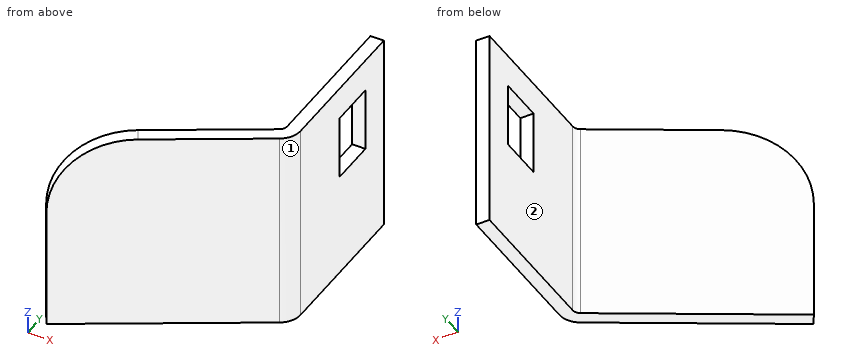
```python
from build123d import *

# Parameters (mm, degrees)
ODGI_CIE_BAZOWE1_DEPTH     = 76
ZAOKR_GLENIE1_R            = 30
WYTNIJ_WYCI_GNI_CIE1_REACH = 120.035
SZKIC2_W                   = 24.223008457
SZKIC2_H                   = 17.102544726


# Sheet-metal steps are written as plain solids
with BuildPart() as part:
    # Szkic1 → Odgięcie bazowe1 (new body)
    with BuildSketch(Plane.XY):
        with BuildLine():
            Line((-70, -40.414518843), (-4, -2.309401077))
            ThreePointArc((-4, -2.309401077), (-1.07179677, 0.618802154), (0, 4.618802154))
            Line((0, 4.618802154), (0, 60))
            Line((0, 60), (-5, 60))
            Line((-5, 60), (-5, 4.618802154))
            ThreePointArc((-5, 4.618802154), (-5.401923789, 3.118802154), (-6.5, 2.020725942))
            Line((-6.5, 2.020725942), (-72.5, -36.084391824))
            Line((-72.5, -36.084391824), (-70, -40.414518843))
        make_face()
    extrude(amount=ODGI_CIE_BAZOWE1_DEPTH)

    # Zaokrąglenie1
    zaokr_glenie1_edges = [part.edges().sort_by_distance(p)[0] for p in [
        (-71.25, -38.249455334, 76),
    ]]
    fillet(zaokr_glenie1_edges, radius=ZAOKR_GLENIE1_R)

    # Szkic2 → Wytnij-wyciągnięcie1 (cut, up to next)
    with BuildSketch(Plane.ZY.offset(5), mode=Mode.PRIVATE) as wytnij_wyci_gni_cie1_sk1:
        with Locations((51.623539351, 39.212758495)):
            Rectangle(SZKIC2_W, SZKIC2_H)
    wytnij_wyci_gni_cie1_tool1 = extrude(wytnij_wyci_gni_cie1_sk1.sketch, amount=-WYTNIJ_WYCI_GNI_CIE1_REACH, mode=Mode.PRIVATE) & part.part
    add(wytnij_wyci_gni_cie1_tool1.solids().sort_by_distance((-5, 39.212758, 51.623539))[0], mode=Mode.SUBTRACT)


solid = part.part
```
Check sheet for the modelled part. Datum: model origin and axes. Units: mm. Face numbers are marked on the shaded views. A direction names the side the tool comes from. Give positions to 0.01 mm unless a question says otherwise; leave off trailing zeros. Write each loop counter-clockwise with the first axis right and the second up, starting at its lowest first coordinate (ties: lowest second). Pieces come first, ordered by that corner, then holes.
Item 1: Scan lines: L1, parallel to X at y = 9, z = 43; L2, parallel to Y at x = -13, z = 61; L3, parallel to X at y = -34, z = 46.5. Record each from-to range of solid material in increasing order.
Item 2: Cross-section at A-A (y = 40). Enter the section's corners in (x, z).
Item 3: Cross-section at B-B (z = 52.5). Enter the section's corners in (x, y), and give its area (3 significant figures).
Item 4: Access from +Z, -Z, +X, -X, +Y, -Y to the whole of each face (thin tool, end or side, straight path). Record for the marked faces 1 and 2.
Item 5: Cross-section at D-D (x = -27). Enter the section's corners in (y, z).
Item 6: Gauge pin test, flat ends, axial feed: pin 1 (3 mm diameter, centred on y = -17, z = 15, fed in from -X); pin 2 (6 mm diameter, centred on x = -45, z = 38.5, fed in from +Y); pin 3 (1 mm diameter, centred on y = 42.5, z = 26.5, fed in from -X). Record the tip position at first contact, or that the pin passes through.
Item 7: Cross-section at C-C (z = 32). Enter the section's corners in (x, y).
Report:
1. L1: x = -5 to 0
1. L2: y = -7.51 to -1.73
1. L3: x = -68.89 to -58.89
2. outline: (-5, 0) - (0, 0) - (0, 39.51) - (-5, 39.51) - close; (-5, 63.74) - (0, 63.74) - (0, 76) - (-5, 76) - close
3. outline: (-71.88, -35.73) - (-69.38, -40.06) - (-4, -2.31) arc R8 ccw to (0, 4.62) - (0, 30.66) - (-5, 30.66) - (-5, 4.62) arc R3 cw to (-6.5, 2.02) - close; (-5, 47.76) - (0, 47.76) - (0, 60) - (-5, 60) - close
3. area: 598 mm2
4. face 1: +Z, -Z, +X, -Y
4. face 2: +Z, -Z, -X, +Y
5. outline: (-15.59, 0) - (-9.81, 0) - (-9.81, 76) - (-15.59, 76) - close
6. pin 1: stops at x = -42.04
6. pin 2: stops at y = -18.48
6. pin 3: stops at x = -5
7. outline: (-72.5, -36.08) - (-70, -40.41) - (-4, -2.31) arc R8 ccw to (0, 4.62) - (0, 60) - (-5, 60) - (-5, 4.62) arc R3 cw to (-6.5, 2.02) - close
